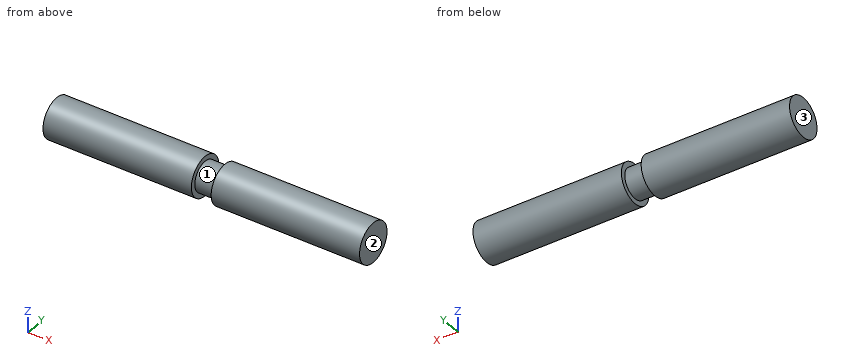
from build123d import *

# Parameters (mm, degrees)
SKETCH3_R           = 6
BOSS_EXTRUDE1_DEPTH = 96
SKETCH4_R           = 7.659234512
SKETCH4_R_2         = 4.5
CUT_EXTRUDE1_DEPTH  = 3


with BuildPart() as part:
    # Sketch3 → Boss-Extrude1 (new body)
    with BuildSketch(Plane(origin=(24, 0, 0), x_dir=(0, 0, -1), z_dir=(1, 0, 0))):
        Circle(SKETCH3_R)
    extrude(amount=-BOSS_EXTRUDE1_DEPTH)

    # Sketch4 → Cut-Extrude1 (cut, symmetric)
    with BuildSketch(Plane(origin=(-24, 0, 0), x_dir=(0, 0, -1), z_dir=(1, 0, 0))):
        Circle(SKETCH4_R)
        Circle(SKETCH4_R_2, mode=Mode.SUBTRACT)
    extrude(amount=CUT_EXTRUDE1_DEPTH, both=True, mode=Mode.SUBTRACT)


solid = part.part
The listing builds one solid part. Answer for the finished solid, in the listing's coordinates (mm). Face numbers are marked on the shaded views. Coordinates: 2 decimals unless noted, no trailing zeros. Order: outer loops, then holes, each group sorted by start corner. A loop starts at its lowest first (then second) coordinate and runs counter-clockwise, first axis right, second up.
Q1. A cutting plane is placed at A-A, the plane z = 0. Write down the section's boundary in (x, y), and give its area (3 significant figures).
Q2. Consider line 1 (X direction, y = -5, z = -0.25); line 2 (Z direction, x = -1, y = 4.25). Determine where each line is inside the solid, lowest interval first.
Q3. Given P1, Ø5, axis at x = -34, z = 3, coming from the -Y side; P2, Ø1.5, axis at x = -29, y = 1, coming from the +Z side; P3, Ø2, axis at x = -56.5, z = -2.5, coming from the -Y side, each flat-ended and moving along its own axis, determine where each tip first touches the part or whether it passes through.
Q4. For a pull along X with two mould halves and no side action, classify the marked faces 1, 2 and 3 as pulls with the +X half, pulls with the -X half, needs draft (parallel to the pull), parting line crosses it, or undercut.
Q5. A cutting plane is placed at C-C, the plane x = -28. Write down the section's boundary in (y, z), and give its area (3 significant figures).
Answers follow:
1. outline: (-72, -6) - (-27, -6) - (-27, -4.5) - (-21, -4.5) - (-21, -6) - (24, -6) - (24, 6) - (-21, 6) - (-21, 4.5) - (-27, 4.5) - (-27, 6) - (-72, 6) - close
1. area: 1,130 mm2
2. line 1: x = -72 to -27, -21 to 24
2. line 2: z = -4.24 to 4.24
3. P1: stops at y = -5.98
3. P2: stops at z = 5.99
3. P3: stops at y = -5.81
4. face 1: undercut
4. face 2: pulls with the +X half
4. face 3: pulls with the -X half
5. outline: circle Ø12 at (0, 0)
5. area: 113 mm2
